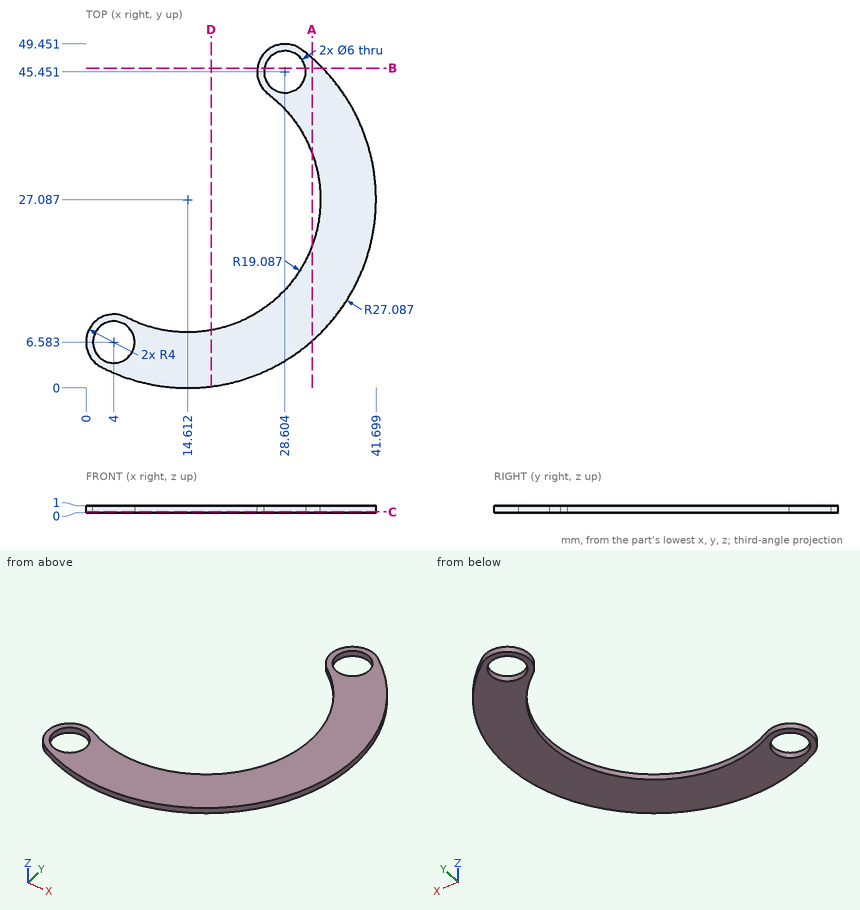
Could you check a few things on this drawing? It's one solid part, dimensions in mm from its lowest x, y, z. Coordinates: 2 decimals unless noted, no trailing zeros. Order: outer loops, then holes, each group sorted by start corner. A loop starts at its lowest first (then second) coordinate and runs counter-clockwise, first axis right, second up.
1. I need wall thicknesses on line 1 (Y direction, x = 4, z = 0.25) (1 decimal); line 2 (Y direction, x = 26, z = 0.6) (1 decimal); line 3 (Y direction, x = 32, z = 0.7) (1 decimal). Which ranges of each line are inside material? Lowest first, please.
2. If we section it at D-D (x = 18): Please give me the cut outline in (y, z).
3. If we section it at A-A (x = 32.5): Please give me the cut outline in (y, z) (1 decimal).
4. If we section it at C-C (z = 0.15): Give the number of separate pieces and of enclosed holes in the cut face, then the cut area to 3 significant figures.
5. If we section it at B-B (y = 46): Please give me the cut outline in (x, z) (1 decimal).
Entries:
1. line 1: y = 2.2 to 3.6, 9.6 to 10.6
1. line 2: y = 2.5 to 11.8, 42.4 to 44, 46.9 to 48.5
1. line 3: y = 6.3 to 19.2, 35 to 47.9
2. outline: (0.21, 0) - (8.3, 0) - (8.3, 1) - (0.21, 1) - close
3. outline: (6.7, 0) - (20.4, 0) - (20.4, 1) - (6.7, 1) - close; (33.7, 0) - (47.4, 0) - (47.4, 1) - (33.7, 1) - close
4. separate pieces: 1
4. enclosed holes: 2
4. area: 542 mm2
5. outline: (24.6, 0) - (25.7, 0) - (25.7, 1) - (24.6, 1) - close; (31.6, 0) - (34, 0) - (34, 1) - (31.6, 1) - close
